Source: CAD feature listing. Evaluate the final solid. Frame: model axes, mm. A direction names the side the tool comes from. Give positions to 0.01 mm unless a question says otherwise; leave off trailing zeros. Loops run counter-clockwise (first coordinate to the right, second up) from the corner with the lowest first, then second, coordinate; pieces in that order, holes last.
```python
from build123d import *

# Parameters (mm, degrees)
F0_R     = 3
F1_DEPTH = 4.15
F2_DEPTH = 60


with BuildPart() as f1:
    # F0 (on Front) → F1 (new body)
    with BuildSketch(Plane.XZ):
        Polygon((2.886751, 5), (-2.886751, 5), (-5.773503, 0), (-2.886751, -5), (2.886751, -5), (5.773503, 0), align=None)
        Circle(F0_R, mode=Mode.SUBTRACT)
        Circle(F0_R)
    extrude(amount=F1_DEPTH)

    # F0 (on Front) → F2 (join)
    with BuildSketch(Plane.XZ):
        Circle(F0_R)
    extrude(amount=F2_DEPTH)


solid = f1.part
```
(1) Section C-C, the plane y = -52. Return the cut outline in (x, z), then the cut area to 3 significant figures.
A:
outline: circle Ø6 at (0, 0)
area: 28.3 mm2
(2) Ray query, line 1 along Y through (x, z) = (3.25, -2); line 2 along X through (y, z) = (-11, 1.25); line 3 along X through (y, z) = (-22, 0.75). Return the intervals inside material, ascending.
A:
line 1: y = -4.15 to 0
line 2: x = -2.73 to 2.73
line 3: x = -2.9 to 2.9
(3) Section A-A, the plane x = 0. Return the cut outline in (y, z).
A:
outline: (-60, -3) - (-4.15, -3) - (-4.15, -5) - (0, -5) - (0, 5) - (-4.15, 5) - (-4.15, 3) - (-60, 3) - close
(4) First-contact query: pin 1 (3 mm diameter, centred on x = 2.5, y = -19.5, fed in from +Z); pin 2 (4 mm diameter, centred on y = -19, z = 3, fed in from -X); pin 3 (1.5 mm diameter, centred on x = 0, y = -45.5, fed in from +Z). Flat tips, straight axial feed; report the tip coordinate or a pass-through.
A:
pin 1: stops at z = 2.83
pin 2: stops at x = -2.83
pin 3: stops at z = 3
(5) Section D-D, the plane x = -4.5. Return the cut outline in (y, z).
A:
outline: (-4.15, -2.21) - (0, -2.21) - (0, 2.21) - (-4.15, 2.21) - close
(6) Section B-B, the plane z = 0.75. Return the cut outline in (x, y), then the cut area to 3 significant figures.
A:
outline: (-5.34, -4.15) - (-2.9, -4.15) - (-2.9, -60) - (2.9, -60) - (2.9, -4.15) - (5.34, -4.15) - (5.34, 0) - (-5.34, 0) - close
area: 369 mm2
(7) Reachability of faces 1 (the flat face through (0, -60, 0)), 2 (the flat face through (2.5, -4.15, 2.3)) from +Z, -Z, +X, -X, +Y, -Y: full face, straight path, thin tool, end or side. Return the list, or none.
A:
face 1: +Z, -Z, +X, -X, -Y
face 2: -Y
